Check sheet for the modelled part. Datum: model origin and axes. Units: mm. Face numbers are marked on the shaded views. A direction names the side the tool comes from. Round coordinates to 2 decimals unless told otherwise and drop trailing zeros. Loops run counter-clockwise (first coordinate to the right, second up) from the corner with the lowest first, then second, coordinate; pieces in that order, holes last. Notation, with made-up numbers: (8.5, 55) - (16.5, 55) arc R26 ccw to (16.5, 93) - close; hole circle Ø8 at (-5, 17). An arc over 180 degrees is marked (long way). Answer in a Markdown table with one row per item. Add a question column.
(1) Gauge pin test, flat ends, axial feed: pin 1 (1.2 mm diameter, centred on x = -4, y = 3.5, fed in from -Z); pin 2 (1.9 mm diameter, centred on x = 0, y = -9, fed in from +Z); pin 3 (1.3 mm diameter, centred on y = -9, z = 1.5, fed in from -X). Record the tip position at first contact, or that the pin passes through.
(2) Mould release check, pull along Y, two halves, no side actions. Record for the marked faces 5, 6 and 7: +Y half, -Y half, draft (parallel to the pull), parting line (faces both ways), or undercut.
(3) Cross-section at C-C on z = 0. Enter the section's corners in (x, y), then the cut area to 3 significant figures.
(4) Access from +Z, -Z, +X, -X, +Y, -Y to the whole of each face (thin tool, end or side, straight path). Record for the marked faces 1, 2, 3 and 4.
(5) Cross-section at A-A on x = 4. Enter the section's corners in (y, z), then the cut area to 3 significant figures.
(6) Cross-section at D-D on x = -3.75. Enter the section's corners in (y, z), then the cut area to 3 significant figures.
(7) Cross-section at B-B on y = -8.25. Enter the section's corners in (x, z).
(8) Thickness scan on line 1 along Y through (x, z) = (-2.25, 1.75); line 2 along X through (y, z) = (2.25, 0); line 3 along X through (y, z) = (2.75, 1.5). Record the ranges inside material, lowest first.
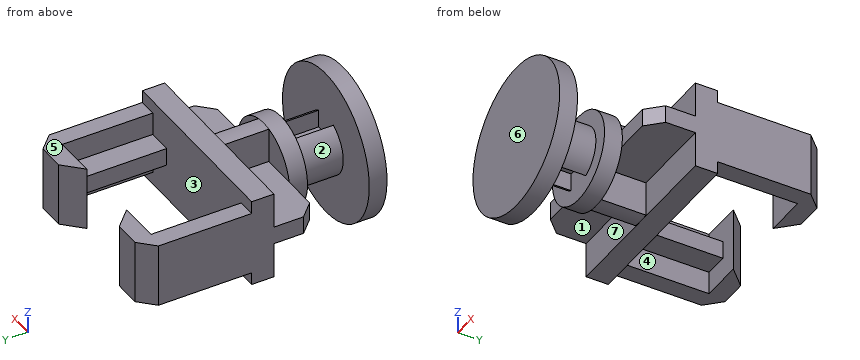
from build123d import *
from build123d.topology import SkipClean

# Parameters (mm, degrees)
SKETCH1_W           = 2.8
SKETCH1_H           = 1.2
SKETCH1_H_2         = 6.1
SKETCH1_H_3         = 4.5
SKETCH1_W_2         = 1.2
SKETCH1_W_3         = 4.6
BOSS_EXTRUDE1_DEPTH = 0.6
BOSS_EXTRUDE2_DEPTH = 1.55
BOSS_EXTRUDE3_DEPTH = 0.85
SKETCH6_R           = 3
BOSS_EXTRUDE4_DEPTH = 1.2
BOSS_EXTRUDE5_START = 3
BOSS_EXTRUDE5_DEPTH = 3
SKETCH8_R           = 2
BOSS_EXTRUDE6_DEPTH = 3
CUT_EXTRUDE1_START  = -3
CUT_EXTRUDE1_DEPTH  = 3
SKETCH10_R          = 5
BOSS_EXTRUDE7_DEPTH = 1.2
CHAMFER1_SIZE       = 1


with BuildPart() as part:
    # Sketch1 → Boss-Extrude1 (new, symmetric)
    with BuildSketch(Plane.XY):
        with Locations((-4.9, 5.3)):
            Rectangle(SKETCH1_W, SKETCH1_H)
        Polygon((-2.3, 4.7), (-3.5, 5.9), (-3.5, 4.7), align=None)
        with Locations((-4.9, 1.65)):
            Rectangle(SKETCH1_W, SKETCH1_H_2)
        with Locations((-4.9, -3.65)):
            Rectangle(SKETCH1_W, SKETCH1_H_3)
        with Locations((-2.9, -3.65)):
            Rectangle(SKETCH1_W_2, SKETCH1_H_3)
        with Locations((0, -3.65)):
            Rectangle(SKETCH1_W_3, SKETCH1_H_3)
        with Locations((2.9, -3.65)):
            Rectangle(SKETCH1_W_2, SKETCH1_H_3)
        with Locations((4.9, -3.65)):
            Rectangle(SKETCH1_W, SKETCH1_H_3)
        with Locations((4.9, 1.65)):
            Rectangle(SKETCH1_W, SKETCH1_H_2)
        Polygon((3.5, 5.9), (2.3, 4.7), (3.5, 4.7), align=None)
        with Locations((4.9, 5.3)):
            Rectangle(SKETCH1_W, SKETCH1_H)
    extrude(amount=BOSS_EXTRUDE1_DEPTH, both=True)

    # Sketch3 → Boss-Extrude2 (add)
    with BuildSketch(Plane.XY.offset(0.6)):
        Polygon((-6.3, 4.7), (-6.3, 5.9), (-5.1, 5.9), (-3.5, 5.9), (-2.3, 4.7), (-3.5, 4.7), (-5.1, 4.7), (-5.1, -1.4), (3.5, -1.4), (5.1, -1.4), (5.115943, 4.7), (3.5, 4.7), (2.3, 4.7), (3.5, 5.9), (6.3, 5.9), (6.3, -2.9), (-6.3, -2.9), align=None)
    boss_extrude2 = extrude(amount=BOSS_EXTRUDE2_DEPTH)

    # Mirror1: Boss-Extrude2 across plane
    add(boss_extrude2.mirror(Plane.XY))

    # Sketch5 → Boss-Extrude3 (add)
    with BuildSketch(Plane(origin=(0, 0, -2.15), x_dir=(-1, 0, 0), z_dir=(0, 0, -1))):
        Polygon((-5.1, -1.4), (-6.3, -1.4), (-6.3, -2.9), (6.3, -2.9), (6.3, -1.4), align=None)
    boss_extrude3 = extrude(amount=BOSS_EXTRUDE3_DEPTH)

    # Mirror2: Boss-Extrude3 across plane
    add(boss_extrude3.mirror(Plane.XY))

    # Sketch6 → Boss-Extrude4 (add)
    with BuildSketch(Plane.XZ.offset(5.9)):
        with Locations(Location((0, 0, 0), (0, 0, 11.536959))):
            Circle(SKETCH6_R)
    extrude(amount=BOSS_EXTRUDE4_DEPTH)

    # Sketch7 → Boss-Extrude5 (add)
    with SkipClean():  # the faces are left unmerged after this step: merging them gives an invalid solid
        with BuildSketch(Plane(origin=(0, -5.9, 0), x_dir=(1, 0, 0), z_dir=(0, 1, 0)).offset(BOSS_EXTRUDE5_START)):
            with BuildLine():
                Line((-0.6, 0.6), (-0.6, -2.939388))
                ThreePointArc((-0.6, -2.939388), (0, -3), (0.6, -2.939388))
                Line((0.6, -2.939388), (0.6, 0.6))
                Line((0.6, 0.6), (-0.6, 0.6))
            make_face()
            with BuildLine():
                Line((-0.6, 2.939388), (-0.6, 0.6))
                Line((-0.6, 0.6), (0.6, 0.6))
                Line((0.6, 0.6), (0.6, 2.939388))
                ThreePointArc((0.6, 2.939388), (0, 3), (-0.6, 2.939388))
            make_face()
        extrude(amount=-BOSS_EXTRUDE5_DEPTH)

    # Sketch8 → Boss-Extrude6 (add)
    with SkipClean():  # the faces are left unmerged after this step: merging them gives an invalid solid
        with BuildSketch(Plane.XZ.offset(7.1)):
            with Locations(Location((0, 0, 0), (0, 0, 270))):
                Circle(SKETCH8_R)
        extrude(amount=BOSS_EXTRUDE6_DEPTH)

    # Sketch9 → Cut-Extrude1 (cut)
    with SkipClean():  # the faces are left unmerged after this step: merging them gives an invalid solid
        with BuildSketch(Plane.XZ.offset(10.1).offset(CUT_EXTRUDE1_START)):
            with BuildLine():
                Line((-0.85, -0.6), (-0.85, -1.810387))
                ThreePointArc((-0.85, -1.810387), (0, -2), (0.85, -1.810387))
                Line((0.85, -1.810387), (0.85, -0.6))
                Line((0.85, -0.6), (-0.85, -0.6))
            make_face()
            with BuildLine():
                ThreePointArc((0.85, 1.810387), (0, 2), (-0.85, 1.810387))
                Line((-0.85, 1.810387), (-0.85, 0.6))
                Line((-0.85, 0.6), (0.85, 0.6))
                Line((0.85, 0.6), (0.85, 1.810387))
            make_face()
        extrude(amount=CUT_EXTRUDE1_DEPTH, mode=Mode.SUBTRACT)

    # Sketch10 → Boss-Extrude7 (add)
    with SkipClean():  # the faces are left unmerged after this step: merging them gives an invalid solid
        with BuildSketch(Plane.XZ.offset(10.1)):
            with Locations(Location((0, 0, 0), (0, 0, 270))):
                Circle(SKETCH10_R)
        extrude(amount=BOSS_EXTRUDE7_DEPTH)

    # Chamfer1
    chamfer1_edges = [part.edges().sort_by_distance(p)[0] for p in [
        (-6.3, 5.9, 0),
        (6.3, 5.9, 0),
        (6.3, -5.9, 0),
        (-6.3, -5.9, 0),
    ]]
    chamfer(chamfer1_edges, length=CHAMFER1_SIZE)


solid = part.part
Answers:
| question | item | result |
|---|---|---|
| 1 | pin 1 | stops at z = -0.6 |
| 1 | pin 2 | stops at z = 1.81 |
| 1 | pin 3 | stops at x = -1.81 |
| 2 | face 5 | draft |
| 2 | face 6 | -Y half |
| 2 | face 7 | undercut |
| 3 | outline | (-6.3, -4.9) - (-5.3, -5.9) - (-3, -5.9) - (-3, -7.1) - (-2, -7.1) - (-2, -10.1) - (-5, -10.1) - (-5, -11.3) - (5, -11.3) - (5, -10.1) - (2, -10.1) - (2, -7.1) - (3, -7.1) - (3, -5.9) - (5.3, -5.9) - (6.3, -4.9) - (6.3, 4.9) - (5.3, 5.9) - (3.5, 5.9) - (2.3, 4.7) - (3.5, 4.7) - (3.5, -1.4) - (-3.5, -1.4) - (-3.5, 4.7) - (-2.3, 4.7) - (-3.5, 5.9) - (-5.3, 5.9) - (-6.3, 4.9) - close |
| 3 | area | 128 mm^2 |
| 4 | face 1 | -Z, -X |
| 4 | face 2 | -X |
| 4 | face 3 | none |
| 4 | face 4 | -Z |
| 5 | outline | (-11.3, -3) - (-10.1, -3) - (-10.1, 3) - (-11.3, 3) - close; (-5.9, -0.6) - (-2.9, -0.6) - (-2.9, -3) - (-1.4, -3) - (-1.4, -0.6) - (4.7, -0.6) - (4.7, -2.15) - (5.9, -2.15) - (5.9, 2.15) - (4.7, 2.15) - (4.7, 0.6) - (-1.4, 0.6) - (-1.4, 3) - (-2.9, 3) - (-2.9, 0.6) - (-5.9, 0.6) - close |
| 5 | area | 32.3 mm^2 |
| 6 | outline | (-11.3, -3.31) - (-10.1, -3.31) - (-10.1, 3.31) - (-11.3, 3.31) - close; (-5.9, -0.6) - (-2.9, -0.6) - (-2.9, -3) - (-1.4, -3) - (-1.4, -0.6) - (4.7, -0.6) - (4.7, -2.15) - (5.9, -2.15) - (5.9, 2.15) - (4.7, 2.15) - (4.7, 0.6) - (-1.4, 0.6) - (-1.4, 3) - (-2.9, 3) - (-2.9, 0.6) - (-5.9, 0.6) - close |
| 6 | area | 33.0 mm^2 |
| 7 | outline | (-0.85, -1.81) - (-0.85, -0.6) - (0.85, -0.6) - (0.85, -1.81) arc R2 ccw to (0.85, 1.81) - (0.85, 0.6) - (-0.85, 0.6) - (-0.85, 1.81) arc R2 ccw to start |
| 8 | line 1 | y = -11.3 to -10.1, -7.1 to -5.9, -2.9 to -1.4 |
| 8 | line 2 | x = -6.3 to -3.5, 3.5 to 6.3 |
| 8 | line 3 | x = -6.3 to -5.1, 5.11 to 6.3 |
